Source: CAD feature listing. Evaluate the final solid. Frame: model axes, mm. Face numbers are marked on the shaded views. A direction names the side the tool comes from. Round coordinates to 2 decimals unless told otherwise and drop trailing zeros. Write each loop counter-clockwise with the first axis right and the second up, starting at its lowest first coordinate (ties: lowest second). Pieces come first, ordered by that corner, then holes. Notation, with made-up numbers: M 22,0.5 L 38,0.5 A17 ccw 38,6.5 Z; hole C 15,49 d2. An arc over 180 degrees is marked long. Use a Markdown table: item, result.
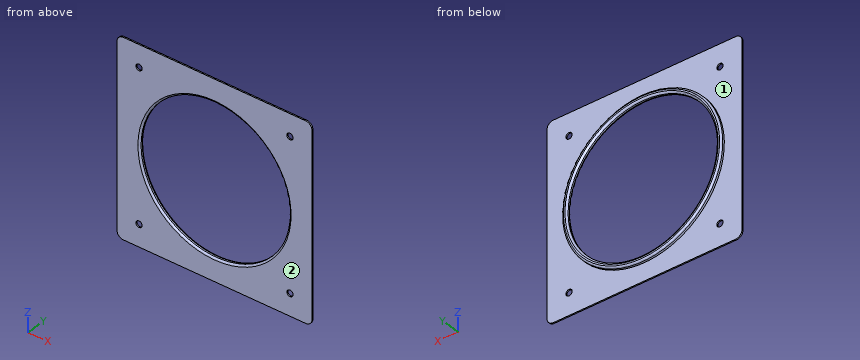
```python
from build123d import *

# Parameters (mm, degrees)
SKETCH1_R           = 59.5
SKETCH1_R_2         = 2.5
BOSS_EXTRUDE1_DEPTH = 1
SKETCH2_R           = 63.5
SKETCH2_R_2         = 59.5
BOSS_EXTRUDE2_DEPTH = 3
FILLET1_R           = 1.4
FILLET2_R           = 1.4


with BuildPart() as part:
    # Sketch1 → Boss-Extrude1 (new body)
    with BuildSketch(Plane(origin=(0, 0, 0), x_dir=(1, 0, 0), z_dir=(0, 1, 0))):
        with BuildLine():
            Line((-72.5, -77.5), (72.5, -77.5))
            ThreePointArc((72.5, -77.5), (76.035533906, -76.035533906), (77.5, -72.5))
            Line((77.5, -72.5), (77.5, 72.5))
            ThreePointArc((77.5, 72.5), (76.035533906, 76.035533906), (72.5, 77.5))
            Line((72.5, 77.5), (-72.5, 77.5))
            ThreePointArc((-72.5, 77.5), (-76.035533906, 76.035533906), (-77.5, 72.5))
            Line((-77.5, 72.5), (-77.5, -72.5))
            ThreePointArc((-77.5, -72.5), (-76.035533906, -76.035533906), (-72.5, -77.5))
        make_face()
        with Locations(Location((0, 0, 0), (0, 0, 270))):
            Circle(SKETCH1_R, mode=Mode.SUBTRACT)
        with Locations(Location((-60, 60, 0), (0, 0, 270))):
            Circle(SKETCH1_R_2, mode=Mode.SUBTRACT)
        with Locations(Location((60, 60, 0), (0, 0, 270))):
            Circle(SKETCH1_R_2, mode=Mode.SUBTRACT)
        with Locations(Location((60, -60, 0), (0, 0, 270))):
            Circle(SKETCH1_R_2, mode=Mode.SUBTRACT)
        with Locations(Location((-60, -60, 0), (0, 0, 270))):
            Circle(SKETCH1_R_2, mode=Mode.SUBTRACT)
    extrude(amount=BOSS_EXTRUDE1_DEPTH)

    # Sketch2 → Boss-Extrude2 (add)
    with BuildSketch(Plane(origin=(0, 1, 0), x_dir=(1, 0, 0), z_dir=(0, 1, 0))):
        with Locations(Location((0, 0, 0), (0, 0, 270))):
            Circle(SKETCH2_R)
        with Locations(Location((0, 0, 0), (0, 0, 270))):
            Circle(SKETCH2_R_2, mode=Mode.SUBTRACT)
    extrude(amount=BOSS_EXTRUDE2_DEPTH)

    # Fillet1
    fillet1_edges = [part.edges().sort_by_distance(p)[0] for p in [
        (0, 4, -63.5),
        (0, 4, -59.5),
    ]]
    fillet(fillet1_edges, radius=FILLET1_R)

    # Fillet2
    fillet2_edges = [part.edges().sort_by_distance(p)[0] for p in [
        (0, 0, -59.5),
    ]]
    fillet(fillet2_edges, radius=FILLET2_R)


solid = part.part
```
Q1. Section D-D on z = -67. Return loops of the section in (x, y).
Results are:
| item | result |
|---|---|
| outline | M -77.5,0 L 77.5,0 L 77.5,1 L -77.5,1 Z |
Q2. Line query: L1, parallel to X at y = 0.45, z = -60; L2, parallel to Y at x = 41.5, z = -68.5; L3, parallel to X at y = 1.1, z = -3.5. Output: solid intervals per line, ascending.
Results are:
| item | result |
|---|---|
| L1 | -77.5 to -62.5, -57.5 to 57.5, 62.5 to 77.5 |
| L2 | 0 to 1 |
| L3 | -63.4 to -59.43, 59.43 to 63.4 |
Q3. Reachability of the marked faces 1 and 2 from +Z, -Z, +X, -X, +Y, -Y: full face, straight path, thin tool, end or side. Return the list, or none.
Results are:
| item | result |
|---|---|
| face 1 | +Y |
| face 2 | +Z, -Z, +X, -X, -Y |
Q4. First-contact query: pin 1 Ø6.5 at (x, z) = (60, -60) entering from +Y; pin 2 Ø3 at (x, z) = (-60, -60) entering from +Y. Flat tips, straight axial feed; report the tip coordinate or a pass-through.
Results are:
| item | result |
|---|---|
| pin 1 | y = 1 |
| pin 2 | through |
Q5. Section A-A on x = 0. Return loops of the section in (y, z).
Results are:
| item | result |
|---|---|
| outline | M 0,-77.5 L 1,-77.5 L 1,-63.5 L 2.6,-63.5 A1.4 ccw 4,-62.1 L 4,-60.9 A1.4 ccw 2.6,-59.5 L 1.4,-59.5 A1.4 ccw 0,-60.9 Z; M 0,60.9 A1.4 ccw 1.4,59.5 L 2.6,59.5 A1.4 ccw 4,60.9 L 4,62.1 A1.4 ccw 2.6,63.5 L 1,63.5 L 1,77.5 L 0,77.5 Z |
Q6. Section B-B on z = 0. Return loops of the section in (x, y).
Results are:
| item | result |
|---|---|
| outline | M -77.5,0 L -60.9,0 A1.4 ccw -59.5,1.4 L -59.5,2.6 A1.4 ccw -60.9,4 L -62.1,4 A1.4 ccw -63.5,2.6 L -63.5,1 L -77.5,1 Z; M 59.5,1.4 A1.4 ccw 60.9,0 L 77.5,0 L 77.5,1 L 63.5,1 L 63.5,2.6 A1.4 ccw 62.1,4 L 60.9,4 A1.4 ccw 59.5,2.6 Z |
Q7. Section C-C on y = 2. Return loops of the section in (x, z).
Results are:
| item | result |
|---|---|
| outline | C 0,0 d127; hole C 0,0 d119 |
